```python
from build123d import *

# Parameters (mm, degrees)
F1_DEPTH = 5
F3_DEPTH = 1.5
F5_DEPTH = 2
F6_R     = 0.5
F7_R     = 0.5
F8_R     = 0.5


with BuildPart() as f1:
    # F0 (on Top) → F1 (new body)
    with BuildSketch(Plane.XY):
        Polygon((-0.55, 0.6), (-0.55, 1.9502386091), (0.55, 1.9502386091), (0.55, 0.6), (2.0002388261, 0.6), (2.55, 0.6), (2.55, 2.9502386091), (0, 2.9502386091), (-2.55, 2.9502386091), (-2.55, 0.6), (-2.0002388261, 0.6), align=None)
    extrude(amount=-F1_DEPTH)



with BuildPart() as f1b:
    # F0 (on Top) → F1, piece 2 (new body)
    with BuildSketch(Plane.XY):
        Polygon((-0.55, -0.6), (-2.0002388261, -0.6), (-2.55, -0.6), (-2.55, -2.9502386091), (0, -2.9502386091), (2.55, -2.9502386091), (2.55, -0.6), (2.0002388261, -0.6), (0.55, -0.6), (0.55, -1.9502386091), (-0.55, -1.9502386091), align=None)
    extrude(amount=-F1_DEPTH)


with BuildPart() as f1_1:
    add(f1.part)

    add(f1b.part)  # F3 merges F1b
    # F2 (on face) → F3 (join)
    with BuildSketch(Plane(origin=(0, 0, -5), x_dir=(1, 0, 0), z_dir=(0, 0, -1))):
        Polygon((0, 1.9502386091), (0, 0), (0, -8), (3, -8), (3, -3.55), (8.0873970663, -3.55), (5.6016603057, 0), (0, 8), (0, 2.9502386091), (2.55, 2.9502386091), (2.55, 0.6), (0.55, 0.6), (0.55, 1.9502386091), align=None)
        Polygon((0, -8), (0, 0), (0, 1.9502386091), (-0.55, 1.9502386091), (-0.55, 0.6), (-2.55, 0.6), (-2.55, 2.9502386091), (0, 2.9502386091), (0, 8), (-5.6016603057, 0), (-8.0873970663, -3.55), (-3, -3.55), (-3, -8), align=None)
        Polygon((-0.55, 1.9502386091), (0, 1.9502386091), (0, 2.9502386091), (-2.55, 2.9502386091), (-2.55, 0.6), (-0.55, 0.6), align=None)
        Polygon((0, 2.9502386091), (0, 1.9502386091), (0.55, 1.9502386091), (0.55, 0.6), (2.55, 0.6), (2.55, 2.9502386091), align=None)
    extrude(amount=F3_DEPTH)

    # F4 (on face) → F5 (join)
    with BuildSketch(Plane.XY.offset(-5)):
        Polygon((3, 8), (-3, 8), (-3, 3.55), (-8.0873970663, 3.55), (0, -8), (8.0873970663, 3.55), (3, 3.55), align=None)
        Polygon((2.3151064033, -2.9502386091), (0, -6.2565532044), (-2.3151064033, -2.9502386091), (-2.55, -2.9502386091), (-2.55, -2.6147757872), (-6.1664149394, 2.55), (-3, 2.55), (-2.55, 2.55), (-2.55, 2.9502386091), (-2, 2.9502386091), (-2, 3.55), (-2, 7), (2, 7), (2, 3.55), (2, 2.9502386091), (2.55, 2.9502386091), (2.55, 2.55), (3, 2.55), (6.1664149394, 2.55), (2.55, -2.6147757872), (2.55, -2.9502386091), align=None, mode=Mode.SUBTRACT)
    extrude(amount=F5_DEPTH)

    # F6
    f6_edges = [f1_1.edges().sort_by_distance(p)[0] for p in [
        (5.543699, 3.55, -6.5),
        (3, 5.775, -6.5),
        (0, 8, -6.5),
        (-3, 5.775, -6.5),
        (-5.543699, 3.55, -6.5),
        (-4.043699, -2.225, -6.5),
        (4.043699, -2.225, -6.5),
    ]]
    fillet(f6_edges, radius=F6_R)

    # F7
    f7_edges = [f1_1.edges().sort_by_distance(p)[0] for p in [
        (4.043699, -2.225, -3),
        (-4.043699, -2.225, -3),
        (-5.543699, 3.55, -3),
        (-3, 5.775, -3),
        (0, 8, -3),
        (3, 5.775, -3),
        (5.543699, 3.55, -3),
    ]]
    fillet(f7_edges, radius=F7_R)

    # F8
    f8_edges = [f1_1.edges().sort_by_distance(p)[0] for p in [
        (-0.55, 1.275119, 0),
        (0, 1.950239, 0),
        (0.55, 1.275119, 0),
        (-0.55, -1.275119, 0),
        (0, -1.950239, 0),
        (0.55, -1.275119, 0),
    ]]
    fillet(f8_edges, radius=F8_R)


solid = f1_1.part
```
The model under review builds one solid part; all positions refer to its coordinate system, in mm. A direction names the side the tool comes from. Round coordinates to 2 decimals unless told otherwise and drop trailing zeros. Loops run counter-clockwise (first coordinate to the right, second up) from the corner with the lowest first, then second, coordinate; pieces in that order, holes last. Notation, with made-up numbers: (38.5, 52.5) -> (44.5, 52.5) arc R27 cw to (44.5, 89.5) -> close; hole circle Ø6 at (-23.75, -7). An arc over 180 degrees is marked (long way). Answer as a JSON object with one key per item and string values. Group by question number.
1) We need section C-C on z = -4.25. Give the number of separate pieces and of enclosed holes in the cut face, then the cut area to 3 significant figures.
2) We need section D-D on z = -5.75. Write out the cut boundary in (x, y), then the cut area to 3 significant figures.
3) For line 1 (Y direction, x = -1.5, z = -4.25); line 2 (X direction, y = 6, z = -4.25); line 3 (Y direction, x = -7, z = -4.5), list the stretches that pass through material, from the lowest coordinate up. Write a range as [from, to].
4) For pin 1 Ø1.1 at (y, z) = (1, -3) entering from -X; pin 2 Ø1 at (x, z) = (2, -2) entering from -Y; pin 3 Ø0.8 at (y, z) = (5.5, -5) entering from +X, all flat-tipped, find the tip position at first contact; note any pin that passes through.
5) We need section B-B on y = 5. Write out the cut boundary in (x, z), then the cut area to 3 significant figures.
6) Mouldability with a two-part tool opening along X and no side actions: class faces 1 (the face through (0, 8, -5)), 2 (the face through (2, 0.6, -2)), 3 (the face through (3, 6, -5)), 4 (the face through (0.55, -1, -3)) as released by +X, released by -X, zero draft, split by the parting line, or undercut.
7) For faces 5 (the face through (1.174, -4.58, -4.014)), 6 (the face through (6, 3.55, -5)), 7 (the face through (-6, 3.55, -5)), list the 3-axis set-ups (+Z, -Z, +X, -X, +Y, -Y) from which the entire face can be reached by the end or side of a thin tool; tool diameter is ignored.
8) We need section A-A on z = -2.75. Write out the cut boundary in (x, y), then the cut area to 3 significant figures.
Result set:
{
 "1": {"separate pieces": "1", "enclosed holes": "3", "area": "68.5 mm²"},
 "2": {"outline": "(-8.09, 3.55) -> (0, -8) -> (8.09, 3.55) -> (3, 3.55) -> (3, 8) -> (-3, 8) -> (-3, 3.55) -> close", "area": "120 mm²"},
 "3": {"line 1": "[-5.86, -4.11], [-2.95, -0.6], [0.6, 2.95], [7, 8]", "line 2": "[-3, -2], [2, 3]", "line 3": "[2, 3.55]"},
 "4": {"pin 1": "x = -6.57", "pin 2": "y = -2.95", "pin 3": "x = 3"},
 "5": {"outline": "(-3, -6) arc R0.5 ccw to (-2.5, -6.5) -> (2.5, -6.5) arc R0.5 ccw to (3, -6) -> (3, -3.5) arc R0.5 ccw to (2.5, -3) -> (2, -3) -> (2, -5) -> (-2, -5) -> (-2, -3) -> (-2.5, -3) arc R0.5 ccw to (-3, -3.5) -> close", "area": "12.8 mm²"},
 "6": {"face 1": "zero draft", "face 2": "undercut", "face 3": "released by +X", "face 4": "undercut"},
 "7": {"face 5": "+Z", "face 6": "+Z, -Z, +X, +Y", "face 7": "+Z, -Z, -X, +Y"},
 "8": {"outline": "(-2.55, -2.95) -> (2.55, -2.95) -> (2.55, -0.6) -> (0.55, -0.6) -> (0.55, -1.95) -> (-0.55, -1.95) -> (-0.55, -0.6) -> (-2.55, -0.6) -> close; (-2.55, 0.6) -> (-0.55, 0.6) -> (-0.55, 1.95) -> (0.55, 1.95) -> (0.55, 0.6) -> (2.55, 0.6) -> (2.55, 2.95) -> (-2.55, 2.95) -> close", "area": "21.0 mm²"}
}
